Geometry check sheet. Reference: the model listing, model coordinates, mm. A direction names the side the tool comes from. Round coordinates to 2 decimals unless told otherwise and drop trailing zeros. Write each loop counter-clockwise with the first axis right and the second up, starting at its lowest first coordinate (ties: lowest second). Pieces come first, ordered by that corner, then holes.
from build123d import *

# Parameters (mm, degrees)
SKETCH1_W                      = 25.65
SKETCH1_H                      = 14
SKETCH1_W_2                    = 14
SKETCH1_H_2                    = 34.73
BOSS_EXTRUDE1_DEPTH            = 42.65
SKETCH2_R                      = 6.425
CUT_EXTRUDE1_DEPTH             = 42.65
SKETCH3_W                      = 1.9
SKETCH3_H                      = 30
CUT_EXTRUDE2_DEPTH             = 42.65
SKETCH4_R                      = 6.425
CUT_EXTRUDE3_DEPTH             = 42.65
SKETCH5_W                      = 32
SKETCH5_H                      = 1.9
CUT_EXTRUDE4_DEPTH             = 42.65
M3_CLEARANCE_HOLE1_D           = 3.6
M3_CLEARANCE_HOLE1_DEPTH       = 10
M3_CLEARANCE_HOLE1_CSINK_D     = 3.65
M3_CLEARANCE_HOLE1_CSINK_ANGLE = 90
M3_CLEARANCE_HOLE1_TIP         = 1.081549114
SKETCH9_W                      = 61.993652624
SKETCH9_H                      = 40.55348858
CUT_EXTRUDE5_DEPTH             = 61.688696641


with BuildPart() as part:
    # Sketch1 → Boss-Extrude1 (new body)
    with BuildSketch(Plane.XY):
        with Locations((-12.825, -7)):
            Rectangle(SKETCH1_W, SKETCH1_H)
        with Locations((7, -17.365)):
            Rectangle(SKETCH1_W_2, SKETCH1_H_2)
    extrude(amount=BOSS_EXTRUDE1_DEPTH)

    # Sketch2 → Cut-Extrude1 (cut)
    with BuildSketch(Plane.XZ.offset(14)):
        with Locations((-14.665, 27.725)):
            Circle(SKETCH2_R)
    extrude(amount=-CUT_EXTRUDE1_DEPTH, mode=Mode.SUBTRACT)

    # Sketch3 → Cut-Extrude2 (cut)
    with BuildSketch(Plane.XZ.offset(14)):
        with Locations((-16.7, 27.65)):
            Rectangle(SKETCH3_W, SKETCH3_H)
    extrude(amount=-CUT_EXTRUDE2_DEPTH, mode=Mode.SUBTRACT)

    # Sketch4 → Cut-Extrude3 (cut)
    with BuildSketch(Plane.ZY):
        with Locations(Location((18.725, -21.745, 0), (0, 0, 270))):
            Circle(SKETCH4_R)
    extrude(amount=-CUT_EXTRUDE3_DEPTH, mode=Mode.SUBTRACT)

    # Sketch5 → Cut-Extrude4 (cut)
    with BuildSketch(Plane.ZY):
        with Locations((26.65, -25.78)):
            Rectangle(SKETCH5_W, SKETCH5_H)
    extrude(amount=-CUT_EXTRUDE4_DEPTH, mode=Mode.SUBTRACT)

    # M3 Clearance Hole1
    with Locations(Plane(origin=(0, 0, 0), x_dir=(-1, 0, 0), z_dir=(0, 0, -1))):
        with Locations((1.1, -5.25), (13.5, -5.25), (-6.99, -21.8)):
            CounterSinkHole(M3_CLEARANCE_HOLE1_D / 2, M3_CLEARANCE_HOLE1_CSINK_D / 2, depth=M3_CLEARANCE_HOLE1_DEPTH, counter_sink_angle=M3_CLEARANCE_HOLE1_CSINK_ANGLE)
            with Locations((0, 0, -(M3_CLEARANCE_HOLE1_DEPTH + M3_CLEARANCE_HOLE1_TIP / 2))):  # 118° drill point
                Cone(0, M3_CLEARANCE_HOLE1_D / 2, M3_CLEARANCE_HOLE1_TIP, mode=Mode.SUBTRACT)

    # Sketch9 → Cut-Extrude5 (cut, through all)
    with BuildSketch(Plane(origin=(0, 0, 0), x_dir=(1, 0, 0), z_dir=(0, 1, 0))):
        with Locations((-5.42180131, -25.55674429)):
            Rectangle(SKETCH9_W, SKETCH9_H)
    extrude(amount=-CUT_EXTRUDE5_DEPTH, mode=Mode.SUBTRACT)


solid = part.part
1. Depth check by flat-ended pin: pin 1 Ø2 at (x, y) = (-13.5, -5.25) entering from +Z; pin 2 Ø1.6 at (x, z) = (-8, 3.5) entering from -Y. Enter the tip coordinate at first touch or a pass-through.
2. Scan lines: line 1 along X through (y, z) = (-5.25, 1.15); line 2 along Y through (x, z) = (-1, 2.2); line 3 along X through (y, z) = (-4, 2.15). Record each from-to range of solid material in increasing order.
3. Release check for a two-part mould opening along Y. For faces 1 (the face through (-1.334, -3.465, 2.689)), 2 (the face through (-25.65, -7, 3)), 3 (the face through (-13, -14, 3)) record: +Y half, -Y half, draft (parallel to the pull), parting line (faces both ways), or undercut.
4. Section check C-C (z = 4.25). Record the cut outline in (x, y).
5. Access from +Z, -Z, +X, -X, +Y, -Y to the whole of each face (thin tool, end or side, straight path). Record for faces 4 (the face through (0, -25, 3)), 5 (the face through (-11.783, -4.709, 2.689)).
6. Section check D-D (x = 6.99). Record the cut outline in (y, z) (3 decimals).
7. Section check A-A (y = -5.25). Record the cut outline in (x, z) (3 decimals), plus the area to 3 significant figures.
8. Section check B-B (y = -21.8). Record the cut outline in (x, z) (3 decimals).
Results below:
1. pin 1: passes through
1. pin 2: stops at y = -14
2. line 1: x = -25.65 to -15.3, -11.7 to -2.9, 0.7 to 14
2. line 2: y = -14 to -7.05, -3.45 to 0
2. line 3: x = -25.65 to -14.8, -12.2 to -2.4, 0.2 to 14
3. face 1: undercut
3. face 2: draft
3. face 3: -Y half
4. outline: (-25.65, -14) - (0, -14) - (0, -34.73) - (14, -34.73) - (14, 0) - (-25.65, 0) - close; hole circle Ø3.6 at (-13.5, -5.25); hole circle Ø3.6 at (-1.1, -5.25); hole circle Ø3.6 at (6.99, -21.8)
5. face 4: +Z, -Z, -X, -Y
5. face 5: +Z, -Z
6. outline: (-34.73, 0) - (-23.625, 0) - (-23.6, 0.025) - (-23.6, 5.28) - (-34.73, 5.28) - close; (-20, 0.025) - (-19.975, 0) - (0, 0) - (0, 5.28) - (-20, 5.28) - close
7. outline: (-25.65, 0) - (-15.325, 0) - (-15.3, 0.025) - (-15.3, 5.28) - (-25.65, 5.28) - close; (-11.7, 0.025) - (-11.675, 0) - (-2.925, 0) - (-2.9, 0.025) - (-2.9, 5.28) - (-11.7, 5.28) - close; (0.7, 0.025) - (0.725, 0) - (14, 0) - (14, 5.28) - (0.7, 5.28) - close
7. area: 171 mm2
8. outline: (0, 0) - (5.165, 0) - (5.19, 0.025) - (5.19, 5.28) - (0, 5.28) - close; (8.79, 0.025) - (8.815, 0) - (14, 0) - (14, 5.28) - (8.79, 5.28) - close
